```python
from build123d import *

# Parameters (mm, degrees)
F2_DEPTH = 3


# Not quite as in the source:
# - a feature names something its author has since deleted; it is built from what else it names


with BuildPart() as f2:
    # F1 (on Top) → F2 (new body)
    with BuildSketch(Plane.XY):
        Polygon((90, 10), (90, 35), (60, 35), (60, 38), (40, 38), (40, 35), (-40, 35), (-40, 38), (-60, 38), (-60, 35), (-90, 35), (-90, 10), (-93, 10), (-93, -10), (-90, -10), (-90, -35), (-60, -35), (-60, -38), (-40, -38), (-40, -35), (40, -35), (40, -38), (60, -38), (60, -35), (90, -35), (90, -10), (93, -10), (93, 10), align=None)
    extrude(amount=F2_DEPTH)


solid = f2.part
```
CAD build for the part. Positions are in the model's coordinates, mm. Give positions to 0.01 mm unless a question says otherwise; leave off trailing zeros. Order: outer loops, then holes, each group sorted by start corner. A loop starts at its lowest first (then second) coordinate and runs counter-clockwise, first axis right, second up. Notation, with made-up numbers: M 50.5,66.25 L 97.5,66.25 A32 ccw 97.5,101.25 Z; hole C -6.75,64.5 d9. An arc over 180 degrees is marked long. Put each result on its own line as item: value. Start each with the question number.
(1) Flat gauge pins, fed straight in: pin 1 Ø1.5 at (y, z) = (-27.5, 1.5) entering from -X; pin 2 Ø8 at (x, y) = (-30, -7.5) entering from -Z; pin 3 Ø0.9 at (y, z) = (-37, 1.5) entering from +X; pin 4 Ø0.9 at (x, z) = (-5, 1.5) entering from -Y. Where does each tip first touch, or does it go through?
(2) Saw through at B-B, the plane y = 23. Write the cut outline in (x, z).
(3) Saw through at A-A, the plane z = 1.6. Write the cut outline in (x, y).
(4) Drill centre lines: line 1 along Y through (x, z) = (14, 0.7); line 2 along X through (y, z) = (-27, 1.1). Where is each one in solid material? Low to high.
(5) Saw through at C-C, the plane x = 33. Write the cut outline in (y, z), then the cut area to 3 significant figures.
Check result:
1. pin 1: stops at x = -90
1. pin 2: stops at z = 0
1. pin 3: stops at x = 60
1. pin 4: stops at y = -35
2. outline: M -90,0 L 90,0 L 90,3 L -90,3 Z
3. outline: M -93,-10 L -90,-10 L -90,-35 L -60,-35 L -60,-38 L -40,-38 L -40,-35 L 40,-35 L 40,-38 L 60,-38 L 60,-35 L 90,-35 L 90,-10 L 93,-10 L 93,10 L 90,10 L 90,35 L 60,35 L 60,38 L 40,38 L 40,35 L -40,35 L -40,38 L -60,38 L -60,35 L -90,35 L -90,10 L -93,10 Z
4. line 1: y = -35 to 35
4. line 2: x = -90 to 90
5. outline: M -35,0 L 35,0 L 35,3 L -35,3 Z
5. area: 210 mm2
